Part model, mm, in its own coordinate system. A direction names the side the tool comes from. Give positions to 0.01 mm unless a question says otherwise; leave off trailing zeros. Order: outer loops, then holes, each group sorted by start corner. A loop starts at its lowest first (then second) coordinate and runs counter-clockwise, first axis right, second up. Notation, with made-up numbers: (14, 34) -> (29, 34) arc R18 cw to (29, 49) -> close; hole circle Ø10 at (23.25, 76.5). An arc over 180 degrees is marked (long way). Write item = value, one per line. Start each with the question number.
Item 1: Flat gauge pins, fed straight in: P1, Ø12.5, axis at y = 22.5, z = 9.5, coming from the +X side; P2, Ø12.5, axis at x = 33.5, z = 15.5, coming from the +Y side; P3, Ø7.5, axis at y = 15.5, z = 13.5, coming from the -X side. Where does each tip first touch, or does it go through?
Item 2: Tool access for faces 1 (the face through (0, 18, 12)), 2 (the face through (61.5, 20, 12)), 3 (the face through (64, 17, 12)), 4 (the face through (-27.15, 36.23, 21.99)): list every direction of +Z, -Z, +X, -X, +Y, -Y with a clear straight run to the whole face (end or side of a thin tool).
Item 3: Band-saw the part on D-D on z = 18. Write the cut outline in (x, y).
Item 4: Band-saw the part on A-A on y = 6. Write the cut outline in (x, z), plus the area to 3 significant figures.
Item 5: Pull direction Z, two halves, no side cores. Call faces 5 (the face through (80.631, 36.268, 10.675)), 6 (the face through (79.3, 35, 9.5)), 7 (the face through (32, 2, 25)): +Z half, -Z half, draft (parallel to the pull), parting line (faces both ways), or undercut.
Item 6: Band-saw the part on B-B on x = -14.25. Write the cut outline in (y, z).
Item 7: Band-saw the part on C-C on z = 12.5. Write the cut outline in (x, y), plus the area to 3 significant figures.
Item 8: Drill centre lines: line 1 along Z through (x, y) = (-14.25, 36.6); line 2 along X through (y, z) = (22, 19); line 3 along Y through (x, z) = (72.5, 18.5). Where is each one in solid material? Low to high.
```python
from build123d import *

# Parameters (mm, degrees)
F1_DEPTH = 25
F2_R     = 10
F3_R     = 1
F4_R     = 3
F5_DEPTH = 25


with BuildPart() as f1:
    # F0 (on Top) → F1 (new body)
    with BuildSketch(Plane.XY):
        Polygon((-30, 37.5), (-30, 35), (0, 35), (0, 0), (64, 0), (64, 35), (94, 35), (94, 37.5), (61.5, 37.5), (61.5, 2.5), (2.5, 2.5), (2.5, 37.5), align=None)
    extrude(amount=F1_DEPTH)

    # F2
    f2_edges = [f1.edges().sort_by_distance(p)[0] for p in [
        (-30, 36.25, 25),
        (-30, 36.25, 0),
        (94, 36.25, 0),
        (94, 36.25, 25),
    ]]
    fillet(f2_edges, radius=F2_R)

    # F3
    f3_edges = [f1.edges().sort_by_distance(p)[0] for p in [
        (64, 35, 12.5),
        (64, 0, 12.5),
        (0, 0, 12.5),
        (0, 35, 12.5),
        (2.5, 37.5, 12.5),
        (2.5, 2.5, 12.5),
        (61.5, 2.5, 12.5),
        (61.5, 37.5, 12.5),
    ]]
    fillet(f3_edges, radius=F3_R)

    # F4 (on face) → F5 (cut)
    with BuildSketch(Plane(origin=(0, 37.5, 0), x_dir=(-1, 0, 0), z_dir=(0, 1, 0))):
        with Locations((14.25, 12.5)):
            Circle(F4_R)
        with Locations((-78.25, 12.5)):
            Circle(F4_R)
    extrude(amount=-F5_DEPTH, mode=Mode.SUBTRACT)


solid = f1.part
```
Values found:
q1.P1 = 64
q1.P2 = 2.5
q1.P3 = 0
q2.face_1 = +Z, -Z, -X, -Y
q2.face_2 = +Z, -Z, +Y
q2.face_3 = +Z, -Z, +X, -Y
q2.face_4 = +Z, -X, +Y, -Y
q3.outline = (-29.54, 35) -> (-1, 35) arc R1 cw to (0, 34) -> (0, 1) arc R1 ccw to (1, 0) -> (63, 0) arc R1 ccw to (64, 1) -> (64, 34) arc R1 cw to (65, 35) -> (93.54, 35) -> (93.54, 37.5) -> (62.5, 37.5) arc R1 ccw to (61.5, 36.5) -> (61.5, 3.5) arc R1 cw to (60.5, 2.5) -> (3.5, 2.5) arc R1 cw to (2.5, 3.5) -> (2.5, 36.5) arc R1 ccw to (1.5, 37.5) -> (-29.54, 37.5) -> close
q4.outline = (0, 0) -> (2.5, 0) -> (2.5, 25) -> (0, 25) -> close; (61.5, 0) -> (64, 0) -> (64, 25) -> (61.5, 25) -> close
q4.area = 125 mm^2
q5.face_5 = undercut
q5.face_6 = draft
q5.face_7 = +Z half
q6.outline = (35, 0) -> (37.5, 0) -> (37.5, 9.5) -> (35, 9.5) -> close; (35, 15.5) -> (37.5, 15.5) -> (37.5, 25) -> (35, 25) -> close
q7.outline = (-30, 35) -> (-17.25, 35) -> (-17.25, 37.5) -> (-30, 37.5) -> close; (-11.25, 35) -> (-1, 35) arc R1 cw to (0, 34) -> (0, 1) arc R1 ccw to (1, 0) -> (63, 0) arc R1 ccw to (64, 1) -> (64, 34) arc R1 cw to (65, 35) -> (75.25, 35) -> (75.25, 37.5) -> (62.5, 37.5) arc R1 ccw to (61.5, 36.5) -> (61.5, 3.5) arc R1 cw to (60.5, 2.5) -> (3.5, 2.5) arc R1 cw to (2.5, 3.5) -> (2.5, 36.5) arc R1 ccw to (1.5, 37.5) -> (-11.25, 37.5) -> close; (81.25, 35) -> (94, 35) -> (94, 37.5) -> (81.25, 37.5) -> close
q7.area = 455 mm^2
q8.line_1 = 0 to 9.5, 15.5 to 25
q8.line_2 = 0 to 2.5, 61.5 to 64
q8.line_3 = 35 to 37.5
